Can you work these out from the model? Positions are in its coordinate system, mm. A direction names the side the tool comes from. Give positions to 0.01 mm unless a question says otherwise; leave off trailing zeros. Order: outer loops, then holes, each group sorted by start corner. A loop starts at its lowest first (then second) coordinate and runs counter-clockwise, first axis right, second up. Notation, with made-up numbers: (25.25, -3.5) - (80.25, -3.5) arc R31 ccw to (80.25, 21.5) - close; hole circle Ø8 at (1, 87). An arc over 180 degrees is marked (long way). Answer as CSV lines item,"result".
Autodesk Fusion 360 part; units mm, degrees
sketch "Boceto1" plane through (0, 0, 0) normal (0, 0, 1) x (1, 0, 0)
  line L0 (0, 0) -> (20, 0)
  line L1 (20, 0) -> (20, 100)
  line L2 (20, 100) -> (0, 100)
  line L3 (0, 100) -> (0, 0)
  dimension "d1" = 20
  dimension "d2" = 100
sketch "Boceto2" plane through (0, 0, 0) normal (1, 0, 0) x (0, 1, 0)
  line L0 (0, 0) -> (100, 0)
  line L1 (100, 0) -> (100, 30)
  line L2 (100, 30) -> (0, 30)
  line L3 (0, 30) -> (0, 0)
  dimension "d3" = 100
  dimension "d4" = 30
sketch "Boceto3" plane through (0, 0, 0) normal (1, 0, 0) x (0, 1, 0)
sketch "Boceto4" plane through (0, 0, 0) normal (0, 1, 0) x (1, 0, 0)
  line L0 (0, 0) -> (20, 0)
  line L1 (20, 0) -> (20, -30)
  line L2 (20, -30) -> (0, -30)
  line L3 (0, -30) -> (0, 0)
  line L4 (0, -30) -> (0, 0)
  dimension "d5" = 20
  dimension "d6" = 30
sketch "Boceto5" plane through (0, 0, 0) normal (0, 0, 1) x (1, 0, 0)
extrude "Extruir1" add sketch "Boceto1" along normal blind 30
sketch "Boceto6" plane through (0, 100, 0) normal (0, 1, 0) x (-1, 0, 0)
  line L0 (-20, 0) -> (0, 0)
  line L1 (0, 0) -> (0, 30)
  line L2 (0, 30) -> (-20, 30)
  line L3 (-20, 30) -> (-20, 0)
  line L4 (-2.5, 2.5) -> (-17.5, 2.5)
  line L5 (-17.5, 2.5) -> (-17.5, 27.5)
  line L6 (-17.5, 27.5) -> (-2.5, 27.5)
  line L7 (-2.5, 27.5) -> (-2.5, 2.5)
  dimension "d9" = 25
  dimension "d10" = 15
extrude "Extruir2" cut sketch "Boceto6" against normal blind 20 contours L4 L5 L6 L7
hole "Agujero1" at (10.0437, 100, 28.1947) direction (0, -1, 0) diameter 1 depth 8 tip angle 118
hole "Agujero2" at (9.9089, 100, 1.7915) direction (0, -1, 0) diameter 1 depth 8 tip angle 118
extrude "Extruir3" cut 1 faces at (7.5, 80, 10.8333) along direction (0, -1, 0) blind 79
extrude "Extruir4" cut 1 faces at (7.5, 1, 10.8333) along direction (0, -1, 0) blind 105
sketch "Boceto7" plane through (20, 0, 0) normal (1, 0, 0) x (0, 1, 0)
  line L0 (0, 0) -> (100, 0)
  line L1 (100, 0) -> (100, 30)
  line L2 (100, 30) -> (0, 30)
  line L3 (0, 30) -> (0, 0)
sketch "Boceto8" plane through (0, 0, 30) normal (0, 0, 1) x (-1, 0, 0)
  line L0 (0, -100) -> (0, 0)
  line L1 (0, 0) -> (-20, 0)
  line L2 (-20, 0) -> (-20, -100)
  line L3 (-20, -100) -> (0, -100)
  line L4 (-20, -100) -> (-20, 0)
  line L5 (-15, -70) -> (-5, -70)
  line L6 (-5, -70) -> (-5, -80)
  line L7 (-5, -80) -> (-15, -80)
  line L8 (-15, -80) -> (-15, -70)
  line L9 (-5, -80) -> (-15, -80)
  line L10 (-15, -80) -> (-15, -70)
  line L11 (-15, -70) -> (-5, -70)
  line L12 (-5, -70) -> (-5, -80)
  dimension "d23" = 100
  dimension "d24" = 20
extrude "Extruir5" cut sketch "Boceto8" against normal blind 7 contours L5 L6 L7 L8 L9 L10 L11 L12
sketch "Boceto9" plane through (0, 0, 30) normal (0, 0, 1) x (-1, 0, 0)
  line L0 (-15, -80) -> (-15, -70)
  line L1 (-15, -70) -> (-5, -70)
  line L2 (-5, -70) -> (-5, -80)
  line L3 (-5, -80) -> (-15, -80)
  line L4 (0, -100) -> (0, 0)
  line L5 (0, 0) -> (-20, 0)
  line L6 (-20, 0) -> (-20, -100)
  line L7 (-20, -100) -> (0, -100)
  line L8 (-15, -80) -> (-5, -80)
  line L9 (-5, -80) -> (-5, -85)
  line L10 (-5, -85) -> (-15, -85)
  line L11 (-15, -85) -> (-15, -80)
extrude "Extruir6" cut sketch "Boceto9" against normal blind 4 contours L3 L8 L9 L10 L11
1) I'm going to push a flat-ended pin straight in: P1, Ø10, axis at x = 2.5, y = 22, coming from the -Z side. Where does the tip first touch, or does it pass through?
Answer block:
P1,"z = 0"
2) If we mould it in two halves opening along Z, with no side actions, what happens to faces 4 (the flat face through (20, 49, 15)), 5 (the flat face through (10, 51, 0)), 6 (the flat face through (17.5, 51, 15))? For each: +Z half, -Z half, draft (parallel to the pull), parting line (faces both ways), or undercut.
Answer block:
face 4,"draft"
face 5,"-Z half"
face 6,"undercut"
3) I want a section at A-A on x = 16.5. Write out the boundary of the cut face in (y, z), plus the area to 3 significant figures.
Answer block:
outline,"(0, 0) - (100, 0) - (100, 2.5) - (0, 2.5) - close; (0, 27.5) - (100, 27.5) - (100, 30) - (0, 30) - close"
area,"500 mm2"
4) I need wall thicknesses on line 1 along X through (y, z) = (9.5, 20); line 2 along Z through (x, y) = (6.25, 13.5). Which ranges of each line are inside material? Lowest first, please. Write a range as [from, to].
Answer block:
line 1,"[0, 2.5], [17.5, 20]"
line 2,"[0, 2.5], [27.5, 30]"
5) I want a section at D-D on x = 7. Write out the boundary of the cut face in (y, z), plus the area to 4 significant figures.
Answer block:
outline,"(0, 0) - (100, 0) - (100, 2.5) - (0, 2.5) - close; (0, 27.5) - (70, 27.5) - (70, 30) - (0, 30) - close; (85, 27.5) - (100, 27.5) - (100, 30) - (85, 30) - close"
area,"462.5 mm2"
6) I want a section at C-C on y = 28. Write out the boundary of the cut face in (x, z).
Answer block:
outline,"(0, 0) - (20, 0) - (20, 30) - (0, 30) - close; hole (2.5, 2.5) - (17.5, 2.5) - (17.5, 27.5) - (2.5, 27.5) - close"
7) Which directions (+Z, -Z, +X, -X, +Y, -Y) give clear straight access to the entire face, cutting with the end or side of a thin tool? Please do faces 1 (the flat face through (10, 70, 29)), 2 (the flat face through (10, 51, 27.5)), 3 (the flat face through (10, 51, 30)).
Answer block:
face 1,"+Z"
face 2,"+Y, -Y"
face 3,"+Z, +X, -X, +Y, -Y"
8) I want a section at B-B on z = 14. Write out the boundary of the cut face in (x, y), plus the area to 3 significant figures.
Answer block:
outline,"(0, 0) - (2.5, 0) - (2.5, 100) - (0, 100) - close; (17.5, 0) - (20, 0) - (20, 100) - (17.5, 100) - close"
area,"500 mm2"
